Geometry: final body of the model. Coordinates: model frame, mm. A direction names the side the tool comes from. Give positions to 0.01 mm unless a question says otherwise; leave off trailing zeros. Write each loop counter-clockwise with the first axis right and the second up, starting at its lowest first coordinate (ties: lowest second). Pieces come first, ordered by that corner, then holes.
Q1. Line query: L1, parallel to Z at x = 65.5, y = -0.5; L2, parallel to Y at x = -38, z = 51.5; L3, parallel to Z at x = -0.5, y = 24.5 (3 decimals). Output: solid intervals per line, ascending.
Q2. Pin query (flat end, axial travel): pin 1 (6 mm diameter, centred on x = 14, z = 37.5, fed in from +Y); pin 2 (10 mm diameter, centred on x = -23, y = 22, fed in from +Z) (3 decimals); pin 3 (1 mm diameter, centred on x = 59, y = -0.5, fed in from +Z). Return the tip coordinate at first contact, or that it passes through.
Q3. Reachability of faces 1 (the face through (66, -25.4, 52)), 2 (the face through (32.73, 16.55, 51.97)), 3 (the face through (103, 0, 49.29)), 4 (the face through (22.225, -17, 18)), 5 (the face through (66, 25.4, 52)) from +Z, -Z, +X, -X, +Y, -Y: full face, straight path, thin tool, end or side. Return the list, or none.
Q4. Cut plane B-B on z = 6. Return the cut outline in (x, y) (3 decimals).
Q5. Cut plane A-A on y = -13. Return the cut outline in (x, z) (3 decimals).
Q6. Cut plane C-C on x = 71. Return the cut outline in (y, z), plus the area to 3 significant figures.
```python
from build123d import *

# Parameters (mm, degrees)
F1_DEPTH = 63.5
F0_W     = 33.928780768
F0_H     = 12.6356402498
F2_DEPTH = 25.4
F3_DEPTH = 7.9375


with BuildPart() as f1:
    # F0 (on Front) → F1 (new body, symmetric)
    with BuildSketch(Plane.XZ):
        Polygon((-41.275, 9.525), (-41.275, -9.525), (41.275, -9.525), (41.275, 9.525), (22.225, 9.525), align=None)
    extrude(amount=F1_DEPTH, both=True)

    # F0 (on Front) → F2 (join, symmetric)
    with BuildSketch(Plane.XZ):
        with BuildLine():
            Line((22.225, 9.525), (41.275, 9.525))
            Line((41.275, 9.525), (41.275, 27.0002))
            ThreePointArc((41.275, 27.0002), (45.9246798487, 38.2255201513), (57.15, 42.8752))
            Line((57.15, 42.8752), (94.253780768, 42.8752))
            Line((94.253780768, 42.8752), (94.253780768, 49.2895597502))
            Line((94.253780768, 49.2895597502), (60.325, 49.2895597502))
            Line((60.325, 49.2895597502), (60.325, 61.9252))
            Line((60.325, 61.9252), (57.15, 61.9252))
            ThreePointArc((57.15, 61.9252), (32.4542956671, 51.6959043329), (22.225, 27.0002))
            Line((22.225, 27.0002), (22.225, 9.525))
        make_face()
        Polygon((60.325, 77.8645597502), (60.325, 61.9252), (94.253780768, 61.9252), (94.253780768, 49.2895597502), (111.125, 49.2895597502), (111.125, 77.8645597502), align=None)
        with Locations((77.289390384, 55.6073798751)):
            Rectangle(F0_W, F0_H)
    extrude(amount=F2_DEPTH, both=True)

    # F0 (on Front) → F3 (join, symmetric)
    with BuildSketch(Plane.XZ):
        with BuildLine():
            add(Edge.make_bspline(
                [(-41.275, 9.525), (-66.8876323333, 38.7312213145), (-87.5999182085, 84.2466196499), (57.15, 61.9252)],
                knots=[0, 0, 0, 0, 111.5045361635, 111.5045361635, 111.5045361635, 111.5045361635], degree=3))
            Line((-41.275, 9.525), (22.225, 9.525))
            Line((22.225, 9.525), (22.225, 27.0002))
            ThreePointArc((22.225, 27.0002), (32.4542956671, 51.6959043329), (57.15, 61.9252))
        make_face()
    extrude(amount=F3_DEPTH, both=True)


solid = f1.part
```
Data:
1. L1: z = 42.88 to 77.86
1. L2: y = -7.94 to 7.94
1. L3: z = -9.525 to 9.525
2. pin 1: stops at y = 7.94
2. pin 2: stops at z = 9.525
2. pin 3: stops at z = 61.93
3. face 1: +Z, +X, -X, -Y
3. face 2: +Z, -X, +Y
3. face 3: -Z, +X, +Y, -Y
3. face 4: +Z, -X, -Y
3. face 5: +Z, +X, -X, +Y
4. outline: (-41.275, -63.5) - (41.275, -63.5) - (41.275, 63.5) - (-41.275, 63.5) - close
5. outline: (-41.275, -9.525) - (41.275, -9.525) - (41.275, 27) arc R15.875 cw to (57.15, 42.875) - (94.254, 42.875) - (94.254, 49.29) - (111.125, 49.29) - (111.125, 77.865) - (60.325, 77.865) - (60.325, 61.925) - (57.15, 61.925) arc R34.925 ccw to (22.225, 27) - (22.225, 9.525) - (-41.275, 9.525) - close
6. outline: (-25.4, 42.88) - (25.4, 42.88) - (25.4, 77.86) - (-25.4, 77.86) - close
6. area: 1,780 mm2
